Could you check a few things on this model? Use its own coordinates, in mm. Give positions to 0.01 mm unless a question says otherwise; leave off trailing zeros. Order: outer loops, then holes, each group sorted by start corner. A loop starts at its lowest first (then second) coordinate and runs counter-clockwise, first axis right, second up. Notation, with made-up numbers: M 79,12.25 L 104,12.25 A28 cw 104,51.25 Z; hole C 37,44 d9. An arc over 180 degrees is marked long. Use a Markdown table: item, result. Add a question column.
Item 1: If we mould it in two halves opening along Z, with no side actions, what happens to faces 1 (the face through (-56.925, 0.022, -59.686)), 2 (the face through (-86, 0, 86)), 3 (the face through (41, 1.588, 41))? For each: released by +Z, released by -Z, zero draft, split by the parting line, or undercut.
Item 2: If I drill on L1, parallel to X at y = 0.85, z = 0; L2, parallel to Z at x = 78, y = -0.3; L3, parallel to X at y = 0.9, z = -55.5, over which ranges is the centre line in solid material (lowest first)? Write a range as from..to.
Item 3: Suppose I cut it at A-A on z = 0. Write out the boundary of the cut face in (x, y), plus the area to 3 significant figures.
Item 4: I'm going to push a flat-ended pin straight in: pin 1 Ø2.5 at (x, z) = (70, -70) entering from +Y. Where does the tip first touch, or does it pass through?
Item 5: Suppose I cut it at D-D on y = 0.35. Count the separate pieces of the cut face and the enclosed holes in it, plus the area to 3 significant figures.
Item 6: Suppose I cut it at C-C on z = -22. Write out the boundary of the cut face in (x, y).
Item 7: Suppose I cut it at B-B on x = 51.5. Write out the boundary of the cut face in (y, z), plus the area to 3 significant figures.
Autodesk Inventor part; units mm, degrees
ref_plane "YZ Plane" through (0, 0, 0) normal (1, 0, 0) x (0, 1, 0)
ref_plane "XZ Plane" through (0, 0, 0) normal (0, 1, 0) x (-1, 0, 0)
ref_plane "XY Plane" through (0, 0, 0) normal (0, 0, 1) x (1, 0, 0)
sketch "Sketch1" plane through (0, 0, 0) normal (0, 1, 0) x (-1, 0, 0)
  line L0 (90, 90) -> (-90, 90)
  line L1 (-90, 90) -> (-90, -90)
  line L2 (-90, -90) -> (90, -90)
  line L3 (90, -90) -> (90, 90)
  line L4 (90, 90) -> (-90, -90) construction
  line L5 (-90, 90) -> (90, -90) construction
  point P0 (0, 0)
  dimension "d0" = 180
  dimension "d1" = 180
extrude "Extrusion1" add sketch "Sketch1" along normal mid plane 3.175
sketch "Sketch2" plane through (0, 1.5875, 0) normal (0, 1, 0) x (1, 0, 0)
  line L0 (90, -90) -> (90, 90) construction
  line L1 (90, 90) -> (-90, 90) construction
  line L2 (-90, 90) -> (-90, -90) construction
  line L3 (-90, -90) -> (90, -90) construction
  circle A0 centre (-64, 64) radius 2.5 construction
  line L4 (0, 90) -> (0, -90) construction
  line L5 (-90, 0) -> (90, 0) construction
  circle A1 centre (-58, 58) radius 2
  circle A2 centre (-58, 70) radius 2
  circle A3 centre (-70, 70) radius 2
  circle A4 centre (-70, 58) radius 2
  circle A5 centre (64, 64) radius 2.5 construction
  circle A6 centre (58, 58) radius 2
  circle A7 centre (58, 70) radius 2
  circle A8 centre (70, 70) radius 2
  circle A9 centre (70, 58) radius 2
  circle A10 centre (-64, -64) radius 2.5 construction
  circle A11 centre (-58, -58) radius 2
  circle A12 centre (-58, -70) radius 2
  circle A13 centre (-70, -70) radius 2
  circle A14 centre (-70, -58) radius 2
  circle A15 centre (64, -64) radius 2.5 construction
  circle A16 centre (58, -58) radius 2
  circle A17 centre (58, -70) radius 2
  circle A18 centre (70, -70) radius 2
  circle A19 centre (70, -58) radius 2
  point P0 (0, 0)
  dimension "d4" = 5
  dimension "d5" = 64
  dimension "d6" = 64
  dimension "d7" = 4
  dimension "d8" = 6
  dimension "d9" = 6
  dimension "d12" = 360
extrude "Extrusion2" cut sketch "Sketch2" against normal through all
chamfer "Chamfer1" distance 8 angle 45 4 edges at (90, 0, 90) (90, 0, -90) (-90, 0, 90) (-90, 0, -90)
sketch "Sketch3" plane through (0, 1.5875, 0) normal (0, 1, 0) x (1, 0, 0)
  circle A0 centre (0, 0) radius 55
  dimension "d19" = 110
extrude "Extrusion3" cut sketch "Sketch3" against normal through all
sketch "Sketch4" plane through (0, 1.5875, 0) normal (0, 1, 0) x (1, 0, 0)
  circle A0 centre (0, 64) radius 7
  circle A1 centre (-32, 55.4256) radius 7
  circle A2 centre (-55.4256, 32) radius 7
  circle A3 centre (-64, 0) radius 7
  circle A4 centre (-55.4256, -32) radius 7
  circle A5 centre (-32, -55.4256) radius 7
  circle A6 centre (0, -64) radius 7
  circle A7 centre (32, -55.4256) radius 7
  circle A8 centre (55.4256, -32) radius 7
  circle A9 centre (64, 0) radius 7
  circle A10 centre (55.4256, 32) radius 7
  circle A11 centre (32, 55.4256) radius 7
  arc A12 (0, 64) -> (-32, 55.4256) centre (0, 0) ccw
  line L0 (-16.5644, 61.8193) -> (0, 0) construction
  circle A13 centre (-16.5644, 61.8193) radius 2
  circle A14 centre (-45.2548, 45.2548) radius 2
  circle A15 centre (-61.8193, 16.5644) radius 2
  circle A16 centre (-61.8193, -16.5644) radius 2
  circle A17 centre (-45.2548, -45.2548) radius 2
  circle A18 centre (-16.5644, -61.8193) radius 2
  circle A19 centre (16.5644, -61.8193) radius 2
  circle A20 centre (45.2548, -45.2548) radius 2
  circle A21 centre (61.8193, -16.5644) radius 2
  circle A22 centre (61.8193, 16.5644) radius 2
  circle A23 centre (45.2548, 45.2548) radius 2
  circle A24 centre (16.5644, 61.8193) radius 2
  dimension "d23" = 14
  dimension "d24" = 64
  dimension "d27" = 360
  dimension "d31" = 4
  dimension "d34" = 360
extrude "Extrusion5" cut sketch "Sketch4" along normal blind 10 and the other way blind 5
sketch "Sketch8" plane through (0, 1.5875, 0) normal (0, 1, 0) x (1, 0, 0)
  circle A0 centre (-78, -86) radius 2
  line L0 (-90, 82) -> (-90, -82)
  line L1 (-82, -90) -> (82, -90)
  circle A1 centre (-46, -86) radius 2
  circle A2 centre (-14, -86) radius 2
  circle A3 centre (86, -78) radius 2
  line L2 (90, -82) -> (90, 82)
  circle A4 centre (86, -46) radius 2
  circle A5 centre (86, -14) radius 2
  circle A6 centre (78, 86) radius 2
  line L3 (82, 90) -> (-82, 90)
  circle A7 centre (46, 86) radius 2
  circle A8 centre (14, 86) radius 2
  circle A9 centre (-86, 78) radius 2
  circle A10 centre (-86, 46) radius 2
  circle A11 centre (-86, 14) radius 2
  circle A12 centre (0, 0) radius 55 construction
  line L4 (0, 55) -> (0, -55) construction
  line L5 (-55, 0) -> (55, 0) construction
  circle A13 centre (78, -86) radius 2
  circle A14 centre (46, -86) radius 2
  circle A15 centre (14, -86) radius 2
  circle A16 centre (86, 78) radius 2
  circle A17 centre (86, 46) radius 2
  circle A18 centre (86, 14) radius 2
  circle A19 centre (-78, 86) radius 2
  circle A20 centre (-46, 86) radius 2
  circle A21 centre (-14, 86) radius 2
  circle A22 centre (-86, -78) radius 2
  circle A23 centre (-86, -46) radius 2
  circle A24 centre (-86, -14) radius 2
  dimension "d63" = 4
  dimension "d65" = 4
  dimension "d68" = 32
  dimension "d73" = 4
  dimension "d74" = 4
  dimension "d75" = 12
  dimension "d78" = 32
  dimension "d85" = 4
  dimension "d86" = 4
  dimension "d87" = 12
  dimension "d90" = 32
  dimension "d97" = 4
  dimension "d98" = 4
  dimension "d99" = 12
  dimension "d102" = 32
  dimension "d109" = 4
extrude "Extrusion8" cut sketch "Sketch8" against normal through all
properties part number "TurretBasePlate"
Findings below:
| question | item | result |
|---|---|---|
| 1 | face 1 | undercut |
| 1 | face 2 | released by +Z |
| 1 | face 3 | zero draft |
| 2 | L1 | x = -90..-71, -57..-55, 55..57, 71..90 |
| 2 | L2 | z = -90..-88, -84..84, 88..90 |
| 2 | L3 | x = -90..-39, -25..25, 39..90 |
| 3 | outline | M -90,-1.59 L -71,-1.59 L -71,1.59 L -90,1.59 Z; M -57,-1.59 L -55,-1.59 L -55,1.59 L -57,1.59 Z; M 55,-1.59 L 57,-1.59 L 57,1.59 L 55,1.59 Z; M 71,-1.59 L 90,-1.59 L 90,1.59 L 71,1.59 Z |
| 3 | area | 133 mm^2 |
| 4 | pin 1 | passes through |
| 5 | separate pieces | 1 |
| 5 | enclosed holes | 65 |
| 5 | area | 20,300 mm^2 |
| 6 | outline | M -90,-1.59 L -50.41,-1.59 L -50.41,1.59 L -90,1.59 Z; M 50.41,-1.59 L 90,-1.59 L 90,1.59 L 50.41,1.59 Z |
| 7 | outline | M -1.59,-90 L 1.59,-90 L 1.59,-37.8 L -1.59,-37.8 Z; M -1.59,-26.2 L 1.59,-26.2 L 1.59,-19.31 L -1.59,-19.31 Z; M -1.59,19.31 L 1.59,19.31 L 1.59,26.2 L -1.59,26.2 Z; M -1.59,37.8 L 1.59,37.8 L 1.59,90 L -1.59,90 Z |
| 7 | area | 375 mm^2 |
